```python
from build123d import *

# Parameters (mm, degrees)
BOSS_EXTRU_1_DEPTH      = 3
ESQUISSE3_W             = 14
ESQUISSE3_H             = 120
ESQUISSE3_W_2           = 16
BOSS_EXTRU_2_DEPTH      = 5
ESQUISSE4_R             = 2.5
ENL_V_MAT_EXTRU_1_DEPTH = 10


with BuildPart() as part:
    # Esquisse2 → Boss.-Extru.1 (new body)
    with BuildSketch(Plane.XY):
        Polygon((0, 0), (175, 0), (175, -120), (142.5, -120), (142.5, -116), (107.5, -116), (107.5, -120), (64.5, -120), (64.5, -116), (29.5, -116), (29.5, -120), (0, -120), align=None)
    extrude(amount=BOSS_EXTRU_1_DEPTH)

    # Esquisse3 → Boss.-Extru.2 (add)
    with BuildSketch(Plane.XY.offset(3)):
        with Locations((19, -60)):
            Rectangle(ESQUISSE3_W, ESQUISSE3_H)
        with Locations((157, -60)):
            Rectangle(ESQUISSE3_W_2, ESQUISSE3_H)
    extrude(amount=-BOSS_EXTRU_2_DEPTH)

    # Esquisse4 → Enlèv. mat.-Extru.1 (cut)
    with BuildSketch(Plane.XY.offset(3)):
        with Locations((47, -107.55)):
            Circle(ESQUISSE4_R)
        with Locations((125, -107.55)):
            Circle(ESQUISSE4_R)
    extrude(amount=-ENL_V_MAT_EXTRU_1_DEPTH, mode=Mode.SUBTRACT)


solid = part.part
```
CAD build for the part. Positions are in the model's coordinates, mm. A direction names the side the tool comes from. Give positions to 0.01 mm unless a question says otherwise; leave off trailing zeros. Write each loop counter-clockwise with the first axis right and the second up, starting at its lowest first coordinate (ties: lowest second). Pieces come first, ordered by that corner, then holes. Notation, with made-up numbers: M -18,40.5 L 25,40.5 A24 cw 25,72.5 Z; hole C 54,3.25 d2. An arc over 180 degrees is marked long. Return JSON: item names as keys, results as strings. Group by question number.
(1) Band-saw the part on B-B (x = 47). Give the cut face in (y, z), and give its area (3 significant figures).
(2) Drill centre lines: L1, parallel to Y at x = 125, z = 1.1; L2, parallel to X at y = -9, z = -1.25; L3, parallel to Z at x = 128.5, y = -44. Where is each one in solid material? Low to high. Write a range as [from, to].
(3) Band-saw the part on C-C (y = -107.55). Give the cut face in (x, z).
(4) Flat gauge pins, fed straight in: pin 1 Ø6.5 at (x, y) = (125, -107.55) entering from +Z; pin 2 Ø1 at (y, z) = (-32.5, -1.5) entering from +X; pin 3 Ø4 at (x, y) = (79.5, -26.5) entering from -Z; pin 4 Ø0.9 at (x, z) = (51, 1.5) entering from -Y. Where does each tip first touch, or does it go through?
(5) 3-axis set-ups, long thin cutter, end or side, ignore diameter. For faces 3 (the face through (170, -59, 0)), 4 (the face through (6, -59, 0)), 5 (the face through (88, -59, 0)): which of +Z, -Z, +X, -X, +Y, -Y reach the whole face in a straight line?
(6) Mould opens along X. For faces 1 (the face through (19, -59, -2)), 2 (the face through (127.385, -106.799, 1.521)) say: pulls with the +X half, pulls with the -X half, needs draft (parallel to the pull), parting line crosses it, or undercut.
(7) Band-saw the part on D-D (y = -51). Give the cut face in (x, z), and give its area (3 significant figures).
(8) Band-saw the part on A-A (z = 0.85). Give the cut face in (x, y), and give its area (3 significant figures).
Entries:
{
 "1": {"outline": "M -116,0 L -110.05,0 L -110.05,3 L -116,3 Z; M -105.05,0 L 0,0 L 0,3 L -105.05,3 Z", "area": "333 mm^2"},
 "2": {"L1": "y = [-116, -110.05], [-105.05, 0]", "L2": "x = [12, 26], [149, 165]", "L3": "z = [0, 3]"},
 "3": {"outline": "M 0,0 L 12,0 L 12,-2 L 26,-2 L 26,0 L 44.5,0 L 44.5,3 L 0,3 Z; M 49.5,0 L 122.5,0 L 122.5,3 L 49.5,3 Z; M 127.5,0 L 149,0 L 149,-2 L 165,-2 L 165,0 L 175,0 L 175,3 L 127.5,3 Z"},
 "4": {"pin 1": "stops at z = 3", "pin 2": "stops at x = 165", "pin 3": "stops at z = 0", "pin 4": "stops at y = -116"},
 "5": {"face 3": "-Z, +X, +Y, -Y", "face 4": "-Z, -X, +Y, -Y", "face 5": "-Z, +Y, -Y"},
 "6": {"face 1": "needs draft", "face 2": "undercut"},
 "7": {"outline": "M 0,0 L 12,0 L 12,-2 L 26,-2 L 26,0 L 149,0 L 149,-2 L 165,-2 L 165,0 L 175,0 L 175,3 L 0,3 Z", "area": "585 mm^2"},
 "8": {"outline": "M 0,-120 L 29.5,-120 L 29.5,-116 L 64.5,-116 L 64.5,-120 L 107.5,-120 L 107.5,-116 L 142.5,-116 L 142.5,-120 L 175,-120 L 175,0 L 0,0 Z; hole C 47,-107.55 d5; hole C 125,-107.55 d5", "area": "20,700 mm^2"}
}
